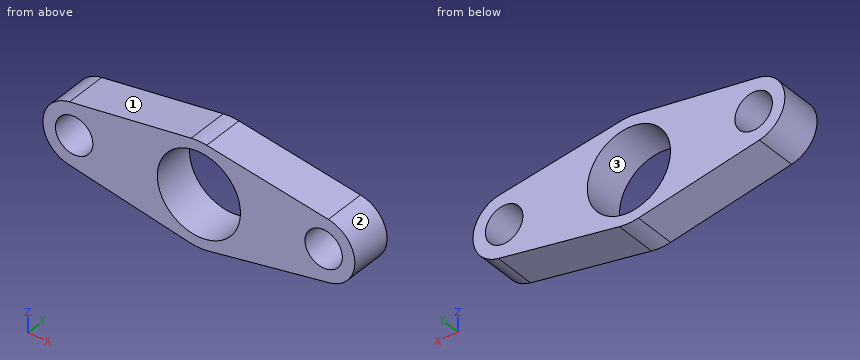
Autodesk Fusion 360 part; units mm, degrees
sketch "Sketch2" plane through (0, 0, 0) normal (0, 1, 0) x (1, 0, 0)
  line L0 (-75, -1.0078) -> (75, -1.0078) construction
  line L1 (3.752, -24.7168) -> (62.2428, -15.8379)
  line L2 (-3.752, -24.7168) -> (-62.2428, -15.8379)
  line L3 (-4.5801, 24.5769) -> (-62.7396, 13.7383)
  line L4 (4.5801, 24.5769) -> (62.7396, 13.7383)
  arc A0 (62.2428, -15.8379) -> (62.7396, 13.7383) centre (59.9915, -1.0078) ccw
  arc A1 (-62.7396, 13.7383) -> (-62.2428, -15.8379) centre (-59.9915, -1.0078) ccw
  arc A2 (-3.752, -24.7168) -> (3.752, -24.7168) centre (0, 0) ccw
  arc A3 (4.5801, 24.5769) -> (-4.5801, 24.5769) centre (0, 0) ccw
  circle A4 centre (0, 0) radius 20
  circle A5 centre (59.9915, -1.0078) radius 9
  circle A6 centre (-59.9915, -1.0078) radius 9
  dimension "d8" = 50
  dimension "d9" = 30
  dimension "d10" = 30
  dimension "d11" = 60
  dimension "d12" = 60
  dimension "d13" = 40
  dimension "d14" = 18
  dimension "d15" = 18
extrude "Extrude1" add sketch "Sketch2" along normal blind 20
Verification items for the finished model (mm, model axes). Face numbers are marked on the shaded views. Coordinates: 2 decimals unless noted, no trailing zeros. Loops run counter-clockwise (first coordinate to the right, second up) from the corner with the lowest first, then second, coordinate; pieces in that order, holes last. Notation, with made-up numbers: (38.25, 79.25) -> (74.25, 79.25) arc R38 cw to (74.25, 117.25) -> close; hole circle Ø7 at (-18, 13.25). An arc over 180 degrees is marked (long way). Answer in a Markdown table with one row per item.
1) Depth check by flat-ended pin: P1, Ø6, axis at x = 35, y = 8, coming from the +Z side; P2, Ø3, axis at y = 17, z = 4, coming from the -X side; P3, Ø8, axis at x = -50.5, y = 11, coming from the +Z side; P4, Ø23.5, axis at x = -59.99, z = 1.01, coming from the -Y side. Enter the tip coordinate at first touch or a pass-through.
The answers:
| item | result |
|---|---|
| P1 | stops at z = 20.43 |
| P2 | stops at x = -74.92 |
| P3 | stops at z = 18.23 |
| P4 | stops at y = 0 |
2) Section check D-D (x = -40.5). Record the cut outline in (y, z).
The answers:
| item | result |
|---|---|
| outline | (0, -17.88) -> (20, -17.88) -> (20, 19.14) -> (0, 19.14) -> close |
3) Section check C-C (y = 2.5). Record the cut outline in (x, z).
The answers:
| item | result |
|---|---|
| outline | (-62.74, -13.74) -> (-4.58, -24.58) arc R25 ccw to (4.58, -24.58) -> (62.74, -13.74) arc R15 ccw to (62.24, 15.84) -> (3.75, 24.72) arc R25 ccw to (-3.75, 24.72) -> (-62.24, 15.84) arc R15 ccw to start; hole circle Ø18 at (-59.99, 1.01); hole circle Ø40 at (0, 0); hole circle Ø18 at (59.99, 1.01) |
4) Draft check along X on the marked faces 1, 2 and 3. Enter one of: released by +X, released by -X, zero draft, split by the parting line, or undercut.
The answers:
| item | result |
|---|---|
| face 1 | released by -X |
| face 2 | released by +X |
| face 3 | undercut |
5) Section check B-B (z = -11.5). Record the cut outline in (x, y).
The answers:
| item | result |
|---|---|
| outline | (-68.27, 0) -> (-16.36, 0) -> (-16.36, 20) -> (-68.27, 20) -> close; (16.36, 0) -> (68.27, 0) -> (68.27, 20) -> (16.36, 20) -> close |
6) Section check A-A (x = 0). Record the cut outline in (y, z), and give its area (3 significant figures).
The answers:
| item | result |
|---|---|
| outline | (0, -25) -> (20, -25) -> (20, -20) -> (0, -20) -> close; (0, 20) -> (20, 20) -> (20, 25) -> (0, 25) -> close |
| area | 200 mm2 |
7) Scan lines: line 1 along X through (y, z) = (6.25, 7.5); line 2 along Z through (x, y) = (-0.5, 19.25); line 3 along X through (y, z) = (15, 0). Record each from-to range of solid material in increasing order. Write a range as from..to.
The answers:
| item | result |
|---|---|
| line 1 | x = -73.51..-66.22, -53.76..-18.54, 18.54..53.76, 66.22..73.51 |
| line 2 | z = -25..-19.99, 19.99..24.99 |
| line 3 | x = -74.96..-68.93, -51.05..-20, 20..51.05, 68.93..74.96 |
